from build123d import *

# Parameters (mm, degrees)
SKETCH2_R           = 75
SKETCH2_R_2         = 59
SKETCH2_R_3         = 46.992946112
BOSS_EXTRUDE1_DEPTH = 6
SKETCH8_R           = 25
CUT_EXTRUDE4_DEPTH  = 6
SKETCH9_R           = 2.5
CUT_EXTRUDE5_DEPTH  = 10


with BuildPart() as part:
    # Sketch1 → Revolve1 (revolve)
    with BuildSketch(Plane(origin=(0, 0, 0), x_dir=(-1, 0, 0), z_dir=(0, 0, -1)), mode=Mode.PRIVATE) as revolve1_sk:
        with BuildLine():
            Line((-59, 0.8724), (-47, 0.8724))
            ThreePointArc((-47, 0.8724), (-46.292893219, 1.165293219), (-46, 1.8724))
            Line((-46, 1.8724), (-46, 5.8724))
            Line((-46, 5.8724), (-47, 6.8724))
            Line((-47, 6.8724), (-49.4043, 6.8724))
            ThreePointArc((-49.4043, 6.8724), (-52.5, 5.8405), (-55.5957, 6.8724))
            Line((-55.5957, 6.8724), (-59, 6.8724))
            Line((-59, 6.8724), (-60, 5.8724))
            Line((-60, 5.8724), (-60, 1.8724))
            ThreePointArc((-60, 1.8724), (-59.707106781, 1.165293219), (-59, 0.8724))
        make_face()
    revolve(revolve1_sk.sketch.rotate(Axis((0, 0, 0), (0, 1, 0)), 270), axis=Axis((0, 0, 0), (0, 1, 0)))

    # Sketch2 → Boss-Extrude1 (add)
    # profile 1 of 2: a face of its own
    with BuildSketch(Plane.XZ.offset(-0.8724)):
        with Locations(Location((0, 0, 0), (0, 0, 270))):
            Circle(SKETCH2_R)
        Circle(SKETCH2_R_2, mode=Mode.SUBTRACT)
    # profile 2 of 2: a face of its own
    with BuildSketch(Plane.XZ.offset(-0.8724)):
        with Locations(Location((0, 0, 0), (0, 0, 270))):
            Circle(SKETCH2_R_3)
    extrude(amount=-BOSS_EXTRUDE1_DEPTH)

    # Sketch8 → Cut-Extrude4 (cut)
    with BuildSketch(Plane(origin=(0, 6.8724, 0), x_dir=(1, 0, 0), z_dir=(0, 1, 0))):
        with Locations(Location((0, 0, 0), (0, 0, 270))):
            Circle(SKETCH8_R)
    extrude(amount=-CUT_EXTRUDE4_DEPTH, mode=Mode.SUBTRACT)

    # Sketch9 → Cut-Extrude5 (cut)
    with BuildSketch(Plane.XZ.offset(-0.8724)):
        with Locations(Location((0, 67.5, 0), (0, 0, 270))):
            Circle(SKETCH9_R)
        with Locations(Location((58.456714755, 33.75, 0), (0, 0, 270))):
            Circle(SKETCH9_R)
        with Locations(Location((58.456714755, -33.75, 0), (0, 0, 270))):
            Circle(SKETCH9_R)
        with Locations(Location((0, -67.5, 0), (0, 0, 270))):
            Circle(SKETCH9_R)
        with Locations(Location((-58.456714755, -33.75, 0), (0, 0, 270))):
            Circle(SKETCH9_R)
        with Locations(Location((-58.456714755, 33.75, 0), (0, 0, 270))):
            Circle(SKETCH9_R)
    extrude(amount=-CUT_EXTRUDE5_DEPTH, mode=Mode.SUBTRACT)


solid = part.part
Can you work these out from the model? Positions are in its coordinate system, mm. Coordinates: 2 decimals unless noted, no trailing zeros. Write each loop counter-clockwise with the first axis right and the second up, starting at its lowest first coordinate (ties: lowest second). Pieces come first, ordered by that corner, then holes.
Q1. Imagine slicing it at B-B, the plane y = 2. List the corners of the cut face in (x, z) for me.
Results found:
outline: circle Ø150 at (0, 0); hole circle Ø5 at (-58.46, -33.75); hole circle Ø5 at (-58.46, 33.75); hole circle Ø50 at (0, 0); hole circle Ø5 at (0, -67.5); hole circle Ø5 at (0, 67.5); hole circle Ø5 at (58.46, -33.75); hole circle Ø5 at (58.46, 33.75)
Q2. Please list where these lines run through material, in increasing order: L1, parallel to Z at x = 12.5, y = 6.75; L2, parallel to Z at x = 60.5, y = 5.5; L3, parallel to X at y = 4.95, z = 0.
Results found:
L1: z = -73.95 to -54, -47.97 to -21.65, 21.65 to 47.97, 54 to 73.95
L2: z = -44.33 to -35.19, -32.31 to 32.31, 35.19 to 44.33
L3: x = -75 to -25, 25 to 75
Q3. Imagine slicing it at D-D, the plane z = 33.75. Count the separate pieces of the cut face and the enclosed holes in it, plus the area to 3 significant figures.
Results found:
separate pieces: 3
enclosed holes: 0
area: 732 mm2
Q4. For P1, Ø1.5, axis at x = -15.5, y = 6, coming from the +Z side; P2, Ø1, axis at y = 4, z = 23.5, coming from the +X side; P3, Ø2, axis at x = 54.5, y = 6, coming from the -Z side, each with a flat end and sliding along its axis, tell me the tip position at first contact or that it passes through.
Results found:
P1: stops at z = 73.54
P2: stops at x = 71.39
P3: stops at z = -52.56
Q5. Imagine slicing it at C-C, the plane z = 67.5. List the corners of the cut face in (x, y) for me, plus the area to 3 significant figures.
Results found:
outline: (-32.69, 0.87) - (-2.5, 0.87) - (-2.5, 6.87) - (-32.69, 6.87) - close; (2.5, 0.87) - (32.69, 0.87) - (32.69, 6.87) - (2.5, 6.87) - close
area: 362 mm2
Q6. If we mould it in two halves opening along Z, with no side actions, what happens to faces 1 (the face through (0.751, 3.83, 65.115)), 2 (the face through (-45.636, 3.83, 59.517)), 3 (the face through (-44, 6.872, -18))? For each: +Z half, -Z half, draft (parallel to the pull), parting line (faces both ways), or undercut.
Results found:
face 1: undercut
face 2: parting line
face 3: draft
